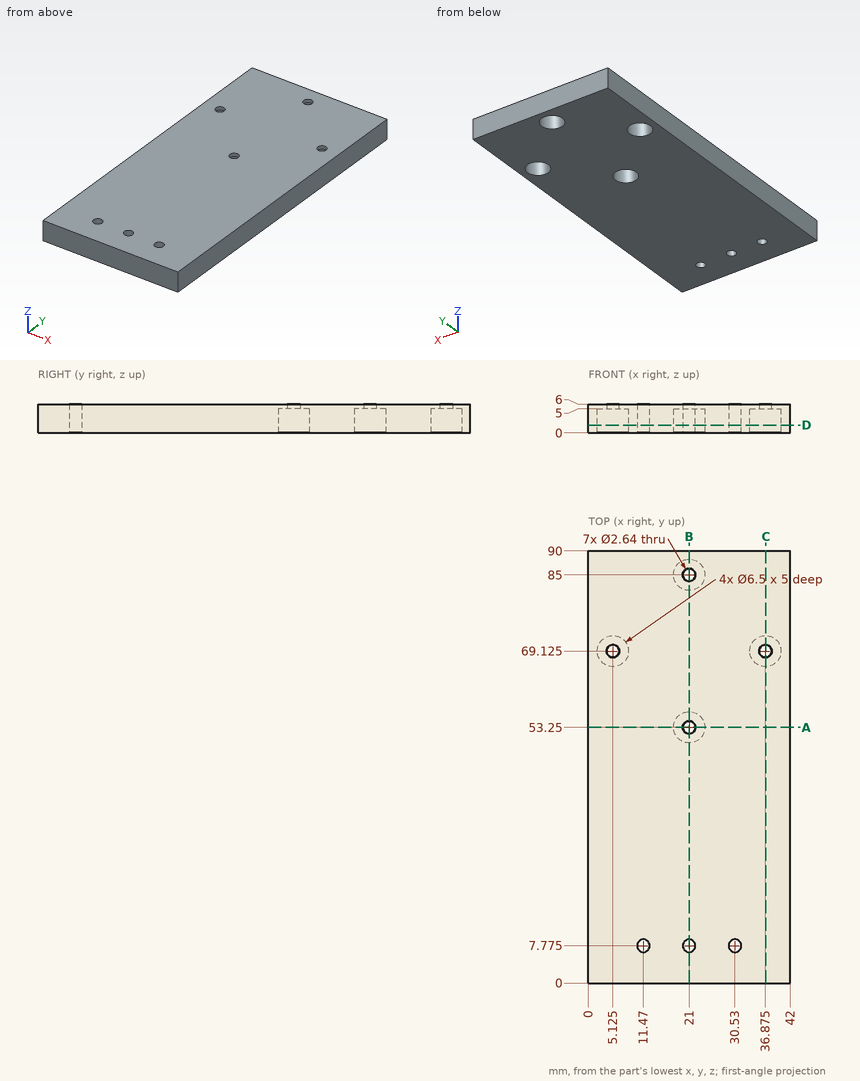
Could you check a few things on this drawing? It's one solid part, dimensions in mm from its lowest x, y, z. Give positions to 0.01 mm unless a question says otherwise; leave off trailing zeros. Write each loop counter-clockwise with the first axis right and the second up, starting at its lowest first coordinate (ties: lowest second). Pieces come first, ordered by that corner, then holes. Notation, with made-up numbers: (58.5, 85.5) -> (104.5, 85.5) arc R19 cw to (104.5, 98.5) -> close; hole circle Ø7 at (20, 76). An arc over 180 degrees is marked (long way). Answer as CSV lines item,"result". Start each with the question number.
(1) If we section it at D-D, the plane z = 1.6: Write out the boundary of the cut face in (x, y) (3 decimals).
(2) Please list where these lines run through material, in increasing order: line 1 (Y direction, x = 21, z = 5.4) (3 decimals); line 2 (X direction, y = 8, z = 5.45); line 3 (Y direction, x = 30.53, z = 3.25) (3 decimals).
(3) If we section it at B-B, the plane x = 21: Write out the boundary of the cut face in (y, z) (3 decimals).
(4) I'm going to push flat-ended pins straight in: pin 1 Ø2.5 at (x, y) = (36.875, 69.125) entering from -Z (1 decimal); pin 2 Ø3 at (x, y) = (5, 68.5) entering from -Z. Where does each tip first touch, or does it pass through?
(5) If we section it at A-A, the plane y = 53.25: Write out the boundary of the cut face in (x, z).
(6) If we section it at C-C, the plane x = 37: Write out the boundary of the cut face in (y, z), and give its area (3 significant figures).
Answer list:
1,outline,"(0, 0) -> (42, 0) -> (42, 90) -> (0, 90) -> close; hole circle Ø6.5 at (5.125, 69.125); hole circle Ø2.64 at (11.47, 7.775); hole circle Ø6.5 at (21, 53.25); hole circle Ø6.5 at (21, 85); hole circle Ø2.64 at (21, 7.775); hole circle Ø2.64 at (30.53, 7.775); hole circle Ø6.5 at (36.875, 69.125)"
2,line 1,"0 to 6.455, 9.095 to 51.93, 54.57 to 83.68, 86.32 to 90"
2,line 2,"0 to 10.17, 12.77 to 19.7, 22.3 to 29.23, 31.83 to 42"
2,line 3,"0 to 6.455, 9.095 to 90"
3,outline,"(0, 0) -> (6.455, 0) -> (6.455, 6) -> (0, 6) -> close; (9.095, 0) -> (50, 0) -> (50, 5) -> (51.93, 5) -> (51.93, 6) -> (9.095, 6) -> close; (54.57, 5) -> (56.5, 5) -> (56.5, 0) -> (81.75, 0) -> (81.75, 5) -> (83.68, 5) -> (83.68, 6) -> (54.57, 6) -> close; (86.32, 5) -> (88.25, 5) -> (88.25, 0) -> (90, 0) -> (90, 6) -> (86.32, 6) -> close"
4,pin 1,"through"
4,pin 2,"z = 5"
5,outline,"(0, 0) -> (17.75, 0) -> (17.75, 5) -> (19.68, 5) -> (19.68, 6) -> (0, 6) -> close; (22.32, 5) -> (24.25, 5) -> (24.25, 0) -> (42, 0) -> (42, 6) -> (22.32, 6) -> close"
6,outline,"(0, 0) -> (65.88, 0) -> (65.88, 5) -> (67.81, 5) -> (67.81, 6) -> (0, 6) -> close; (70.44, 5) -> (72.37, 5) -> (72.37, 0) -> (90, 0) -> (90, 6) -> (70.44, 6) -> close"
6,area,"505 mm^2"
